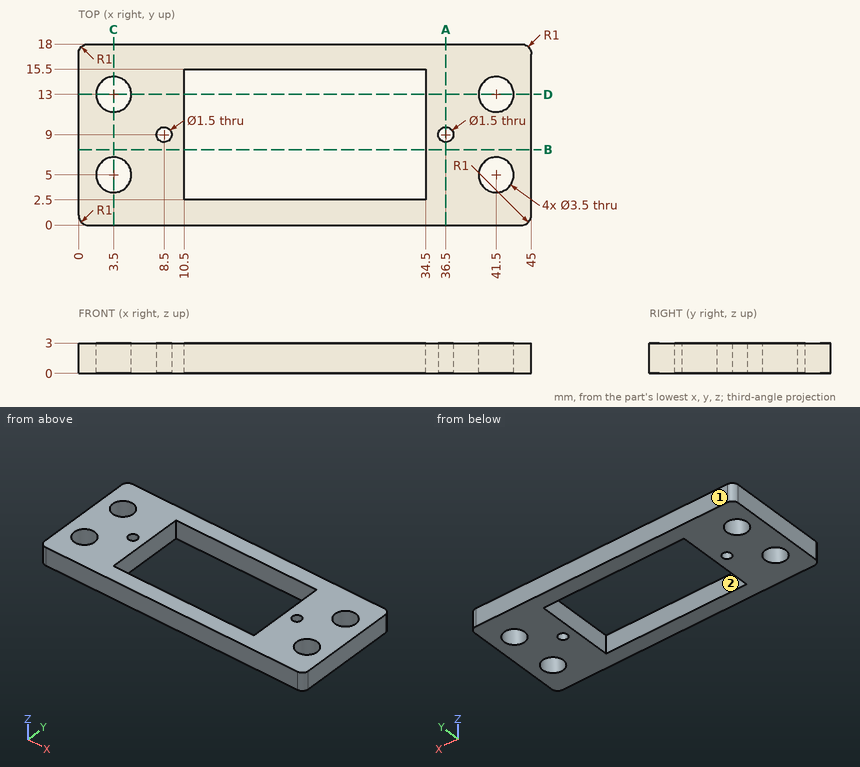
Geometry: see drawing. Coordinates: mm, zero at the bounding-box minimum. Give positions to 0.01 mm unless a question says otherwise; leave off trailing zeros. Write each loop counter-clockwise with the first axis right and the second up, starting at its lowest first coordinate (ties: lowest second). Pieces come first, ordered by that corner, then holes. Notation, with made-up numbers: M -18,-0.5 L 27,-0.5 A24 ccw 27,9.5 Z; hole C -33,-28.5 d4. An arc over 180 degrees is marked long. Answer as a JSON object with one key per item and string values.
Q1. Cut plane C-C, the plane x = 3.5. Return the cut outline in (y, z).
Geometry check:
{"outline": "M 0,0 L 3.25,0 L 3.25,3 L 0,3 Z; M 6.75,0 L 11.25,0 L 11.25,3 L 6.75,3 Z; M 14.75,0 L 18,0 L 18,3 L 14.75,3 Z"}
Q2. Mould query, pull axis X, two halves, no side actions, for the marked faces 1 and 2. Classes: +X half, -X half, draft (parallel to the pull), parting line (faces both ways), or undercut.
Geometry check:
{"face 1": "draft", "face 2": "undercut"}
Q3. Cut plane B-B, the plane y = 7.5. Return the cut outline in (x, z).
Geometry check:
{"outline": "M 0,0 L 10.5,0 L 10.5,3 L 0,3 Z; M 34.5,0 L 45,0 L 45,3 L 34.5,3 Z"}
Q4. Ray query, line 1 along X through (y, z) = (5, 1.7); line 2 along Y through (x, z) = (3.5, 2.3); line 3 along X through (y, z) = (10, 2.5). Return the intervals inside material, ascending.
Geometry check:
{"line 1": "x = 0 to 1.75, 5.25 to 10.5, 34.5 to 39.75, 43.25 to 45", "line 2": "y = 0 to 3.25, 6.75 to 11.25, 14.75 to 18", "line 3": "x = 0 to 10.5, 34.5 to 45"}
Q5. Cut plane D-D, the plane y = 13. Return the cut outline in (x, z), then the cut area to 3 significant figures.
Geometry check:
{"outline": "M 0,0 L 1.75,0 L 1.75,3 L 0,3 Z; M 5.25,0 L 10.5,0 L 10.5,3 L 5.25,3 Z; M 34.5,0 L 39.75,0 L 39.75,3 L 34.5,3 Z; M 43.25,0 L 45,0 L 45,3 L 43.25,3 Z", "area": "42.0 mm^2"}
Q6. Contact query for a flat-ended pin moving along its axis: P1, Ø4, axis at x = 41.5, y = 5, coming from the -Z side. Output: stop coordinate, or through.
Geometry check:
{"P1": "stops at z = 0"}
Q7. Cut plane A-A, the plane x = 36.5. Return the cut outline in (y, z), then the cut area to 3 significant figures.
Geometry check:
{"outline": "M 0,0 L 8.25,0 L 8.25,3 L 0,3 Z; M 9.75,0 L 18,0 L 18,3 L 9.75,3 Z", "area": "49.5 mm^2"}
